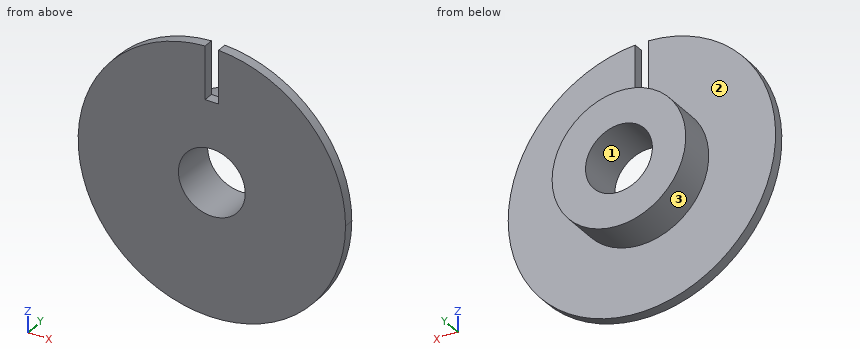
```python
from build123d import *

# Parameters (mm, degrees)
F0_R     = 10
F0_R_2   = 5
F1_DEPTH = 5.5
F2_R     = 20
F2_R_2   = 5
F3_DEPTH = 1.5
F4_W     = 2
F4_H     = 10
F5_DEPTH = 1.501


with BuildPart() as f1:
    # F0 (on Front) → F1 (new body)
    with BuildSketch(Plane.XZ):
        Circle(F0_R)
        Circle(F0_R_2, mode=Mode.SUBTRACT)
    extrude(amount=-F1_DEPTH)

    # F2 (on Front) → F3 (join)
    with BuildSketch(Plane.XZ):
        Circle(F2_R)
        Circle(F2_R_2, mode=Mode.SUBTRACT)
    extrude(amount=F3_DEPTH)

    # F4 (on Front) → F5 (cut, through all)
    with BuildSketch(Plane.XZ):
        with Locations((0, 17)):
            Rectangle(F4_W, F4_H)
    extrude(amount=F5_DEPTH, mode=Mode.SUBTRACT)


solid = f1.part
```
Can you work these out from the model? Positions are in its coordinate system, mm. Face numbers are marked on the shaded views. Coordinates: 2 decimals unless noted, no trailing zeros. Loops run counter-clockwise (first coordinate to the right, second up) from the corner with the lowest first, then second, coordinate; pieces in that order, holes last. Notation, with made-up numbers: M -9.75,59 L 37.25,59 A20 ccw 37.25,75 Z; hole C 69,-30 d7. An arc over 180 degrees is marked long. Put each result on its own line as item: value. Start each with the question number.
(1) I need wall thicknesses on probe 1 along Z at (x, y) = (0, 2.25); probe 2 along Y at (x, z) = (-15, 6); probe 3 along X at (y, z) = (3.5, -2). Which ranges of each line are inside material? Lowest first, please.
(2) Imagine slicing it at D-D on z = -3.5. List the corners of the cut face in (x, y) for me.
(3) Imagine slicing it at B-B on x = 0. List the corners of the cut face in (y, z) for me, and give its area (3 significant figures).
(4) Will these pins go through, and if not, where does the flat tip stop? pin 1 Ø1.6 at (y, z) = (-0.5, 15.5) entering from +X; pin 2 Ø4 at (x, z) = (12, 11.5) entering from +Y; pin 3 Ø0.8 at (x, y) = (-0.5, -1) entering from +Z.
(5) Imagine slicing it at A-A on z = 16. List the corners of the cut face in (x, y) for me, and give its area (3 significant figures).
(6) Imagine slicing it at C-C on y = 0.5. List the corners of the cut face in (x, z) for me.
(7) We'd pull the mould along X, two halves only. Please class the marked faces 1, 2 and 3: +X half, -X half, draft (parallel to the pull), parting line (faces both ways), or undercut.
Worked answers:
1. probe 1: z = -10 to -5, 5 to 10
1. probe 2: y = -1.5 to 0
1. probe 3: x = -9.8 to -4.58, 4.58 to 9.8
2. outline: M -19.69,-1.5 L -3.57,-1.5 L -3.57,5.5 L -9.37,5.5 L -9.37,0 L -19.69,0 Z; M 3.57,-1.5 L 19.69,-1.5 L 19.69,0 L 9.37,0 L 9.37,5.5 L 3.57,5.5 Z
3. outline: M -1.5,-20 L 0,-20 L 0,-10 L 5.5,-10 L 5.5,-5 L -1.5,-5 Z; M -1.5,5 L 5.5,5 L 5.5,10 L 0,10 L 0,12 L -1.5,12 Z
3. area: 88.0 mm2
4. pin 1: stops at x = 13.56
4. pin 2: stops at y = 0
4. pin 3: stops at z = 12
5. outline: M -12,-1.5 L -1,-1.5 L -1,0 L -12,0 Z; M 1,-1.5 L 12,-1.5 L 12,0 L 1,0 Z
5. area: 33.0 mm2
6. outline: C 0,0 d20; hole C 0,0 d10
7. face 1: undercut
7. face 2: draft
7. face 3: parting line
